Here's how the part is built. I have some questions about the finished solid (model axes, mm). Face numbers are marked on the shaded views. A direction names the side the tool comes from. Round coordinates to 2 decimals unless told otherwise and drop trailing zeros. Write each loop counter-clockwise with the first axis right and the second up, starting at its lowest first coordinate (ties: lowest second). Pieces come first, ordered by that corner, then holes. Notation, with made-up numbers: (-17.5, 44.25) -> (13.5, 44.25) arc R16 ccw to (13.5, 48.25) -> close; hole circle Ø3 at (28.25, -36). An arc over 180 degrees is marked (long way). Answer in a Markdown table with one row per item. Add a question column.
Autodesk Inventor part; units mm, degrees
ref_plane "YZ Plane" through (0, 0, 0) normal (1, 0, 0) x (0, 1, 0)
ref_plane "XZ Plane" through (0, 0, 0) normal (0, 1, 0) x (-1, 0, 0)
ref_plane "XY Plane" through (0, 0, 0) normal (0, 0, 1) x (1, 0, 0)
sketch "Sketch1" plane through (0, 0, 0) normal (0, 1, 0) x (-1, 0, 0)
  circle A0 centre (0, 0) radius 11.25
  circle A1 centre (0, 0) radius 17.5
  dimension "d0" = 22.5
  dimension "d1" = 35
extrude "Extrusion1" add sketch "Sketch1" along normal blind 8
sketch "Sketch2" plane through (0, 8, 0) normal (0, 1, 0) x (1, 0, 0)
  circle A0 centre (0, 0) radius 17.5
  circle A1 centre (0, 0) radius 8.9803
extrude "Extrusion2" add sketch "Sketch2" along normal blind 9.525
sketch "Sketch3" plane through (0, 17.525, 0) normal (0, 1, 0) x (1, 0, 0)
  circle A0 centre (0, 0) radius 17.5
  line L0 (-17.5, 0) -> (-17.5, 23.6629)
  line L1 (-17.5, 23.6629) -> (17.5, 23.6629)
  line L2 (17.5, 23.6629) -> (17.5, 0)
  arc A1 (-17.5, 0) -> (17.5, 0) centre (0, 0) ccw
extrude "Extrusion3" add sketch "Sketch3" along normal blind 3
properties part number "hubholder"
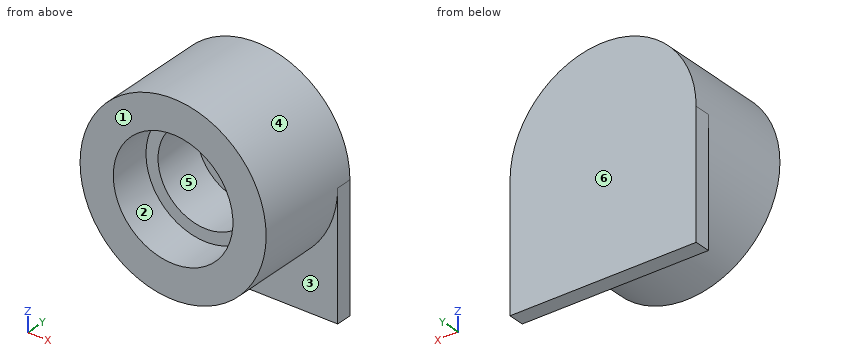
Item 1: If we section it at C-C on y = 10.25: Please give me the cut outline in (x, z).
Item 2: If we mould it in two halves opening along X, with no side actions, what happens to the marked faces 4, 5 and 6? For each: pulls with the +X half, pulls with the -X half, needs draft (parallel to the pull), parting line crosses it, or undercut.
Item 3: On a 3-axis mill with a long thin cutter (end or side, diameter ignored), from which of +Z, -Z, +X, -X, +Y, -Y can I reach the whole of each face in a straight line? I mean the marked faces 1, 2 and 3. Say none if no direction works.
Item 4: For P1, Ø16, axis at x = 0, z = 0, coming from the -Y side (3 decimals); P2, Ø1.5, axis at x = 1, z = -8.5, coming from the -Y side; P3, Ø2, axis at y = 10.5, z = -6.5, coming from the +X side, each with a flat end and sliding along its axis, tell me the tip position at first contact or that it passes through.
Item 5: I need wall thicknesses on line 1 along X through (y, z) = (12.25, 0); line 2 along X through (y, z) = (1, 0.5). Which ranges of each line are inside material? Lowest first, please. Write a range as from..to.
Item 6: If we section it at A-A on y = 5.5: Please give me the cut outline in (x, z).
Item 7: If we section it at B-B on y = 19.5: Please give me the cut outline in (x, z).
Results list:
| question | item | result |
|---|---|---|
| 1 | outline | circle Ø35 at (0, 0); hole circle Ø17.96 at (0, 0) |
| 2 | face 4 | parting line crosses it |
| 2 | face 5 | undercut |
| 2 | face 6 | needs draft |
| 3 | face 1 | +Z, -Z, +X, -X, -Y |
| 3 | face 2 | -Y |
| 3 | face 3 | -Z, -Y |
| 4 | P1 | y = 17.525 |
| 4 | P2 | y = 8 |
| 4 | P3 | x = 16.61 |
| 5 | line 1 | -17.5..-8.98, 8.98..17.5 |
| 5 | line 2 | -17.49..-11.24, 11.24..17.49 |
| 6 | outline | circle Ø35 at (0, 0); hole circle Ø22.5 at (0, 0) |
| 7 | outline | (-17.5, -23.66) -> (17.5, -23.66) -> (17.5, 0) arc R17.5 ccw to (-17.5, 0) -> close |
